Input: part model. Units: mm. Frame: model coordinates. A direction names the side the tool comes from. Give positions to 0.01 mm unless a question says otherwise; leave off trailing zeros. Write each loop counter-clockwise with the first axis right and the second up, starting at its lowest first coordinate (ties: lowest second). Pieces come first, ordered by that corner, then holes. Notation, with made-up numbers: (88, 18) - (120, 18) arc R13 cw to (120, 23) - close; hole circle Ø1 at (-30.5, 85.25). An arc over 180 degrees is marked (long way). Use a Markdown table: item, result. Add a question column.
1. Material intervals for probe 1 along X at (y, z) = (20, -97); probe 2 along Y at (x, z) = (12, -69); probe 3 along Z at (x, y) = (-13, -51.5), sorted ascending.
2. Set-up query: faces 1 (the flat face through (0, -41, -9)), 2 (the cylindrical face through (0, -75, -97)), 3 (the cylindrical face through (32.992, 20.852, -97.042)), 4 (the flat face through (-7.9, -3.3, -94)). Return all of +Z, -Z, +X, -X, +Y, -Y with unobstructed straight access to the full face (end or side cutting, diameter ignored); none if empty.
3. Pin query (flat end, axial travel): pin 1 (4 mm diameter, centred on x = -3.5, z = -44.5, fed in from -Y); pin 2 (19 mm diameter, centred on y = -23, z = -60, fed in from -X); pin 3 (1.5 mm diameter, centred on x = -10.5, y = 22.5, fed in from +Z). Return the tip coordinate at first contact, or that it passes through.
4. Section query B-B, the plane x = 0. Return loops of the section in (y, z), plus the area to 3 significant figures.
5. Section query A-A, the plane y = 20.5. Return loops of the section in (x, z).
6. Section query C-C, the plane z = 0. Return loops of the section in (x, y), plus the area to 3 significant figures.
7. Section query D-D, the plane x = 25. Return loops of the section in (y, z), plus the area to 3 significant figures.
8. Mould query, pull axis Z, two halves, no side actions, for faces 5 (the flat face through (13, 3, -57)), 6 (the flat face through (-26.376, -32.635, -97.042)), 7 (the flat face through (1, -3, -100)). Classes: released by +Z, released by -Z, zero draft, split by the parting line, or undercut.
```python
from build123d import *

# Parameters (mm, degrees)
SKETCH1_R           = 18
BOSS_EXTRUDE1_DEPTH = 41
SKETCH3_R           = 6
BOSS_EXTRUDE2_DEPTH = 6
SKETCH4_W           = 81
SKETCH4_H           = 82
BOSS_EXTRUDE3_DEPTH = 3
SKETCH6_R           = 22
BOSS_EXTRUDE4_DEPTH = 6
BOSS_EXTRUDE5_START = -6
SKETCH7_R           = 22
BOSS_EXTRUDE5_DEPTH = 6
BOSS_EXTRUDE6_DEPTH = 3
HOLE1_D             = 16
HOLE1_DEPTH         = 6


with BuildPart() as part:
    # Sketch1 → Boss-Extrude1 (new, symmetric)
    with BuildSketch(Plane(origin=(0, 0, 0), x_dir=(1, 0, 0), z_dir=(0, 1, 0))):
        with Locations(Location((0, 0, 0), (0, 0, 270))):
            Circle(SKETCH1_R)
    extrude(amount=BOSS_EXTRUDE1_DEPTH, both=True)



with BuildPart() as body_2:
    # Sketch3 → Boss-Extrude2 (new body)
    with BuildSketch(Plane.XY.offset(-100)):
        with BuildLine():
            Line((-38, 41), (38, 41))
            Line((38, 41), (38, 0))
            Line((38, 0), (15.072405416, -64.368667895))
            ThreePointArc((15.072405416, -64.368667895), (0, -75), (-15.072405416, -64.368667895))
            Line((-15.072405416, -64.368667895), (-38, 0))
            Line((-38, 0), (-38, 41))
        make_face()
        with Locations((0, -59)):
            Circle(SKETCH3_R, mode=Mode.SUBTRACT)
    extrude(amount=BOSS_EXTRUDE2_DEPTH)


with BuildPart() as part_1:
    add(part.part)

    add(body_2.part)  # Boss-Extrude3 merges body 2
    # Sketch4 → Boss-Extrude3 (add, symmetric)
    with BuildSketch(Plane(origin=(0, 0, 0), x_dir=(0, 0, -1), z_dir=(1, 0, 0))):
        with Locations((53.5, 0)):
            Rectangle(SKETCH4_W, SKETCH4_H)
    extrude(amount=BOSS_EXTRUDE3_DEPTH, both=True)

    # Sketch6 → Boss-Extrude4 (add)
    with BuildSketch(Plane(origin=(0, 41, 0), x_dir=(1, 0, 0), z_dir=(0, 1, 0))):
        Circle(SKETCH6_R)
    extrude(amount=-BOSS_EXTRUDE4_DEPTH)

    # Sketch7 → Boss-Extrude5 (add)
    with BuildSketch(Plane.XZ.offset(41).offset(BOSS_EXTRUDE5_START)):
        Circle(SKETCH7_R)
    extrude(amount=BOSS_EXTRUDE5_DEPTH)

    # Sketch8 → Boss-Extrude6 (add, symmetric)
    with BuildSketch(Plane(origin=(0, 0, 0), x_dir=(1, 0, 0), z_dir=(0, 1, 0))):
        with BuildLine():
            Line((-28, 94), (-17.900985099, -1.885399817))
            ThreePointArc((-17.900985099, -1.885399817), (0, 18), (17.900985099, -1.885399817))
            Line((17.900985099, -1.885399817), (28, 94))
            Line((28, 94), (-28, 94))
        make_face()
    extrude(amount=BOSS_EXTRUDE6_DEPTH, both=True)

    # Hole1
    with Locations(Plane.XY.offset(-94)):
        with Locations((25, 20.5), (-25, 20.5)):
            Hole(HOLE1_D / 2, depth=HOLE1_DEPTH)


solid = part_1.part
```
Result sheet:
| question | item | result |
|---|---|---|
| 1 | probe 1 | x = -38 to -32.98, -17.02 to 17.02, 32.98 to 38 |
| 1 | probe 2 | y = -3 to 3 |
| 1 | probe 3 | z = -100 to -94 |
| 2 | face 1 | +Z, +X, -X, -Y |
| 2 | face 2 | +Z, -Z, -Y |
| 2 | face 3 | -Z |
| 2 | face 4 | none |
| 3 | pin 1 | stops at y = -41 |
| 3 | pin 2 | stops at x = -3 |
| 3 | pin 3 | stops at z = 15.13 |
| 4 | outline | (-75, -100) - (-65, -100) - (-65, -94) - (-75, -94) - close; (-53, -100) - (41, -100) - (41, 22) - (35, 22) - (35, 18) - (-35, 18) - (-35, 22) - (-41, 22) - (-41, -94) - (-53, -94) - close |
| 4 | area | 9,860 mm² |
| 5 | outline | (-38, -100) - (-33, -100) - (-33, -94) - (-38, -94) - close; (-17, -100) - (17, -100) - (17, -94) - (3, -94) - (3, -17.75) arc R18 ccw (long way) to (-3, -17.75) - (-3, -94) - (-17, -94) - close; (33, -100) - (38, -100) - (38, -94) - (33, -94) - close |
| 6 | outline | (-22, -41) - (22, -41) - (22, -35) - (18, -35) - (18, -3) - (18.1, -3) - (18.1, 3) - (18, 3) - (18, 35) - (22, 35) - (22, 41) - (-22, 41) - (-22, 35) - (-18, 35) - (-18, 3) - (-18.1, 3) - (-18.1, -3) - (-18, -3) - (-18, -35) - (-22, -35) - close |
| 6 | area | 3,050 mm² |
| 7 | outline | (-36.5, -100) - (12.5, -100) - (12.5, -94) - (3, -94) - (3, -65.52) - (-3, -65.52) - (-3, -94) - (-36.5, -94) - close; (28.5, -100) - (41, -100) - (41, -94) - (28.5, -94) - close |
| 7 | area | 540 mm² |
| 8 | face 5 | undercut |
| 8 | face 6 | zero draft |
| 8 | face 7 | released by -Z |
